Could you check a few things on this model? Use its own coordinates, in mm. Face numbers are marked on the shaded views. Round coordinates to 2 decimals unless told otherwise and drop trailing zeros. Loops run counter-clockwise (first coordinate to the right, second up) from the corner with the lowest first, then second, coordinate; pieces in that order, holes last. Notation, with made-up numbers: (57.25, 43) -> (77.25, 43) arc R10 ccw to (77.25, 54) -> close; hole circle Ø5 at (2, -33.5). An arc over 180 degrees is marked (long way). Write each question's results on one line, items separated by ' | '.
from build123d import *

# Parameters (mm, degrees)
FILLET1_R = 1.2


with BuildPart() as part:
    # Sketch1 → Revolve1 (revolve)
    with BuildSketch(Plane.XY, mode=Mode.PRIVATE) as revolve1_sk:
        with BuildLine():
            Line((0, 0), (0, 53))
            ThreePointArc((0, 53), (3.514718626, 61.485281374), (12, 65))
            Line((12, 65), (120, 65))
            ThreePointArc((120, 65), (123.467838025, 64.48799806), (126.63975275, 62.995683239))
            Line((126.63975275, 62.995683239), (156.485534451, 43.170263967))
            ThreePointArc((156.485534451, 43.170263967), (159.128796722, 41.926668283), (162.018661743, 41.5))
            Line((162.018661743, 41.5), (166, 41.5))
            Line((166, 41.5), (166, 46.5))
            Line((166, 46.5), (178, 46.5))
            Line((178, 46.5), (178, 0))
            Line((178, 0), (0, 0))
        make_face()
    revolve(revolve1_sk.sketch.rotate(Axis((0, 0, 0), (1, 0, 0)), 90), axis=Axis((0, 0, 0), (1, 0, 0)))

    # Fillet1
    fillet1_edges = [part.edges().sort_by_distance(p)[0] for p in [
        (178, 0, -46.5),
        (166, 0, -46.5),
    ]]
    fillet(fillet1_edges, radius=FILLET1_R)


solid = part.part
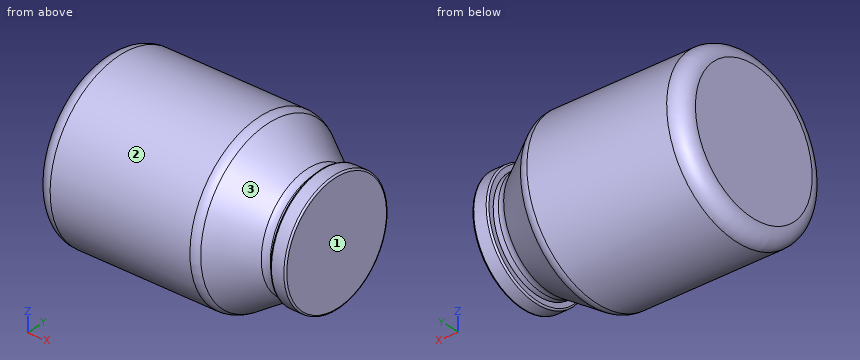
1) If we mould it in two halves opening along X, with no side actions, what happens to the marked faces 1, 2 and 3? For each: released by +X, released by -X, zero draft, split by the parting line, or undercut.
Model answer:
face 1: released by +X | face 2: zero draft | face 3: undercut
2) I want a section at D-D, the plane x = 143. Write out the boundary of the cut face in (y, z), plus the area to 3 significant figures.
Model answer:
outline: circle Ø104.26 at (0, 0) | area: 8,540 mm2
3) I need wall thicknesses on line 1 (X direction, y = -9, z = -41.5); line 2 (Z direction, x = 163.5, y = 8); line 3 (X direction, y = 47.5, z = -38.5). Which ranges of each line are inside material? Lowest first, please.
Model answer:
line 1: x = 0 to 157.73, 166 to 178 | line 2: z = -40.72 to 40.72 | line 3: x = 3.19 to 129.43
4) I'm going to push flat-ended pins straight in: pin 1 (6 mm diameter, centred on x = 49.5, z = 33, fed in from +Y); pin 2 (6 mm diameter, centred on x = 46, z = -31, fed in from -Y); pin 3 (10 mm diameter, centred on x = 87.5, z = 9, fed in from +Y). Where does each tip first touch, or does it pass through?
Model answer:
pin 1: stops at y = 57.66 | pin 2: stops at y = -58.66 | pin 3: stops at y = 64.88
5) I want a section at A-A, the plane y = 0. Write out the boundary of the cut face in (x, z).
Model answer:
outline: (0, -53) arc R12 ccw to (12, -65) -> (120, -65) arc R12 ccw to (126.64, -63) -> (156.49, -43.17) arc R10 cw to (162.02, -41.5) -> (166, -41.5) -> (166, -45.3) arc R1.2 ccw to (167.2, -46.5) -> (176.8, -46.5) arc R1.2 ccw to (178, -45.3) -> (178, 45.3) arc R1.2 ccw to (176.8, 46.5) -> (167.2, 46.5) arc R1.2 ccw to (166, 45.3) -> (166, 41.5) -> (162.02, 41.5) arc R10 cw to (156.49, 43.17) -> (126.64, 63) arc R12 ccw to (120, 65) -> (12, 65) arc R12 ccw to (0, 53) -> close
6) I want a section at C-C, the plane x = 79. Write out the boundary of the cut face in (y, z), plus the area to 3 significant figures.
Model answer:
outline: circle Ø130 at (0, 0) | area: 13,300 mm2
